from build123d import *

# Parameters (mm, degrees)
SKETCH1_W             = 200
SKETCH1_H             = 82.6
BASE_FLANGE1_DEPTH    = 2
SKETCH6_R             = 2
CUT_EXTRUDE1_DEPTH    = 148.587569056
SKETCH7_R             = 12
CUT_EXTRUDE2_DEPTH    = 148.587569056
SKETCH8_R             = 2
SKETCH8_W             = 63
SKETCH8_H             = 67.6
CUT_EXTRUDE3_DEPTH    = 148.587569056
CHAMFER1_SIZE         = 1
SKETCH10_W            = 82.6
SKETCH10_H            = 2
BOSS_EXTRUDE1_DEPTH   = 12
SKETCH11_W            = 82.6
SKETCH11_H            = 2
BOSS_EXTRUDE2_DEPTH   = 12
SKETCH12_W            = 12
SKETCH12_H            = 67.6
CUT_EXTRUDE4_DEPTH    = 159.943577694
FILLET2_R             = 2.5
F_3_0MM_DOWEL_HOLE1_D = 3


# Sheet-metal steps are written as plain solids
with BuildPart() as part:
    # Sketch1 → Base-Flange1 (new body)
    with BuildSketch(Plane(origin=(0, 0, 0), x_dir=(1, 0, 0), z_dir=(0, 1, 0))):
        with Locations((39.040431267, 8.155525606)):
            Rectangle(SKETCH1_W, SKETCH1_H)
    extrude(amount=-BASE_FLANGE1_DEPTH)

    # Sketch6 → Cut-Extrude1 (cut, through all)
    with BuildSketch(Plane(origin=(0, 0, 0), x_dir=(1, 0, 0), z_dir=(0, 1, 0))):
        with Locations(Location((-56.959568733, 45.455525606, 0), (0, 0, 270))):
            Circle(SKETCH6_R)
        with Locations(Location((-56.959568733, -29.144474394, 0), (0, 0, 270))):
            Circle(SKETCH6_R)
        with Locations(Location((135.040431267, -29.144474394, 0), (0, 0, 270))):
            Circle(SKETCH6_R)
        with Locations(Location((135.040431267, 45.455525606, 0), (0, 0, 270))):
            Circle(SKETCH6_R)
    extrude(amount=-CUT_EXTRUDE1_DEPTH, mode=Mode.SUBTRACT)

    # Sketch7 → Cut-Extrude2 (cut, through all)
    with BuildSketch(Plane(origin=(0, 0, 0), x_dir=(1, 0, 0), z_dir=(0, 1, 0))):
        with Locations(Location((39.040431267, 8.155525606, 0), (0, 0, 270))):
            Circle(SKETCH7_R)
    extrude(amount=-CUT_EXTRUDE2_DEPTH, mode=Mode.SUBTRACT)

    # Sketch8 → Cut-Extrude3 (cut, through all)
    with BuildSketch(Plane(origin=(0, 0, 0), x_dir=(1, 0, 0), z_dir=(0, 1, 0))):
        with Locations(Location((17.040431267, 30.155525606, 0), (0, 0, 270))):
            Circle(SKETCH8_R)
        with Locations(Location((61.040431267, 30.155525606, 0), (0, 0, 270))):
            Circle(SKETCH8_R)
        with Locations(Location((61.040431267, -13.844474394, 0), (0, 0, 270))):
            Circle(SKETCH8_R)
        with Locations(Location((17.040431267, -13.844474394, 0), (0, 0, 270))):
            Circle(SKETCH8_R)
        with Locations((-21.959568733, 8.155525606)):
            Rectangle(SKETCH8_W, SKETCH8_H)
        with Locations((100.040431267, 8.155525606)):
            Rectangle(SKETCH8_W, SKETCH8_H)
    extrude(amount=-CUT_EXTRUDE3_DEPTH, mode=Mode.SUBTRACT)

    # Chamfer1
    chamfer1_edges = [part.edges().sort_by_distance(p)[0] for p in [
        (135.040431267, -2, -47.455525606),
        (135.040431267, -2, 27.144474394),
        (-56.959568733, -2, 27.144474394),
        (-56.959568733, -2, -47.455525606),
        (17.040431267, -2, 11.844474394),
        (61.040431267, -2, 11.844474394),
        (61.040431267, -2, -32.155525606),
        (17.040431267, -2, -32.155525606),
    ]]
    chamfer(chamfer1_edges, length=CHAMFER1_SIZE)

    # Sketch10 → Boss-Extrude1 (add)
    with BuildSketch(Plane.ZY.offset(60.959568733)):
        with Locations((-8.155525606, -1)):
            Rectangle(SKETCH10_W, SKETCH10_H)
    extrude(amount=BOSS_EXTRUDE1_DEPTH)

    # Sketch11 → Boss-Extrude2 (add)
    with BuildSketch(Plane(origin=(139.040431267, 0, 0), x_dir=(0, 0, -1), z_dir=(1, 0, 0))):
        with Locations((8.155525606, -1)):
            Rectangle(SKETCH11_W, SKETCH11_H)
    extrude(amount=BOSS_EXTRUDE2_DEPTH)

    # Sketch12 → Cut-Extrude4 (cut, through all)
    with BuildSketch(Plane(origin=(0, 0, 0), x_dir=(1, 0, 0), z_dir=(0, 1, 0))):
        with Locations((-59.459568733, 8.155525606)):
            Rectangle(SKETCH12_W, SKETCH12_H)
        with Locations((137.540431267, 8.155525606)):
            Rectangle(SKETCH12_W, SKETCH12_H)
    extrude(amount=-CUT_EXTRUDE4_DEPTH, mode=Mode.SUBTRACT)

    # Fillet2
    fillet2_edges = [part.edges().sort_by_distance(p)[0] for p in [
        (-72.959568733, -1, 33.144474394),
        (-72.959568733, -1, -49.455525606),
        (151.040431267, -1, 33.144474394),
        (151.040431267, -1, -49.455525606),
        (-65.459568733, -1, 25.644474394),
        (-65.459568733, -1, -41.955525606),
        (143.540431267, -1, -41.955525606),
        (143.540431267, -1, 25.644474394),
        (68.540431267, -1, 25.644474394),
        (68.540431267, -1, -41.955525606),
        (9.540431267, -1, -41.955525606),
        (9.540431267, -1, 25.644474394),
    ]]
    fillet(fillet2_edges, radius=FILLET2_R)

    # Ø3.0mm Dowel Hole1 (through all)
    with Locations(Plane(origin=(0, -2, 0), x_dir=(-1, 0, 0), z_dir=(0, -1, 0))):
        with Locations((69.7595751, -29.944469865), (69.759567513, 46.255524386), (-21.840432167, 46.255524386), (-21.84042458, -29.944469865), (-56.240437954, 46.255521078), (-56.240430367, -29.944473174), (-147.840430047, -29.944473174), (-147.840437634, 46.255521078)):
            Hole(F_3_0MM_DOWEL_HOLE1_D / 2)


solid = part.part
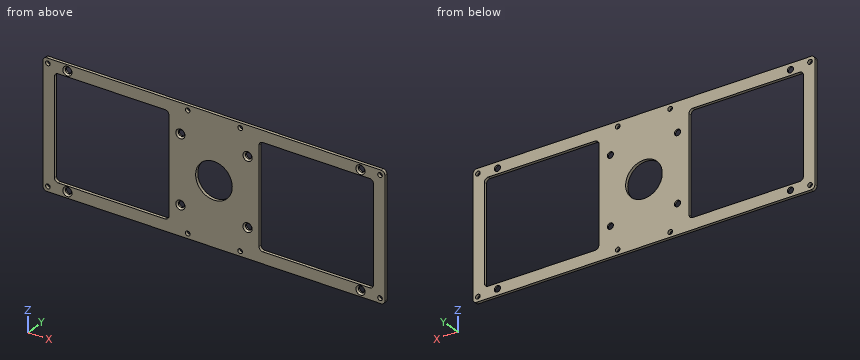
Could you check a few things on this model? Use its own coordinates, in mm. Round coordinates to 2 decimals unless told otherwise and drop trailing zeros. Write each loop counter-clockwise with the first axis right and the second up, starting at its lowest first coordinate (ties: lowest second). Pieces come first, ordered by that corner, then holes. Notation, with made-up numbers: (68.25, -20) -> (74.25, -20) arc R14 cw to (74.25, -16) -> close; hole circle Ø8 at (-33.75, 59.25). An arc over 180 degrees is marked (long way). Use a Markdown table: item, result.
1. If we section it at D-D (x = 32.5): List the corners of the cut face in (y, z) for me, then the cut area to 3 significant figures.
Answer key:
| item | result |
|---|---|
| outline | (-2, -49.46) -> (0, -49.46) -> (0, -18.22) -> (-2, -18.22) -> close; (-2, 1.91) -> (0, 1.91) -> (0, 33.14) -> (-2, 33.14) -> close |
| area | 125 mm^2 |
2. Please list where these lines run through material, in increasing order: probe 1 along X at (y, z) = (-0.65, -23.5); probe 2 along Z at (x, y) = (107, -1.35); probe 3 along X at (y, z) = (-1.15, -31).
Answer key:
| item | result |
|---|---|
| probe 1 | x = -72.96 to -65.46, 9.54 to 68.54, 143.54 to 151.04 |
| probe 2 | z = -49.46 to -41.96, 25.64 to 33.14 |
| probe 3 | x = -72.96 to -65.46, 9.54 to 15.06, 19.02 to 59.06, 63.02 to 68.54, 143.54 to 151.04 |
3. If we section it at A-A (z = 20.5): List the corners of the cut face in (x, y) for me, then the cut area to 3 significant figures.
Answer key:
| item | result |
|---|---|
| outline | (-72.96, -2) -> (-65.46, -2) -> (-65.46, 0) -> (-72.96, 0) -> close; (9.54, -2) -> (68.54, -2) -> (68.54, 0) -> (9.54, 0) -> close; (143.54, -2) -> (151.04, -2) -> (151.04, 0) -> (143.54, 0) -> close |
| area | 148 mm^2 |
4. If we section it at C-C (y = -0.5): State how many separate pieces and enclosed holes the cut face has, then the cut area to 3 significant figures.
Answer key:
| item | result |
|---|---|
| separate pieces | 1 |
| enclosed holes | 19 |
| area | 7,760 mm^2 |
5. If we section it at B-B (x = -1): List the corners of the cut face in (y, z) for me, then the cut area to 3 significant figures.
Answer key:
| item | result |
|---|---|
| outline | (-2, -49.46) -> (0, -49.46) -> (0, -41.96) -> (-2, -41.96) -> close; (-2, 25.64) -> (0, 25.64) -> (0, 33.14) -> (-2, 33.14) -> close |
| area | 30.0 mm^2 |
